from build123d import *

# Parameters (mm, degrees)
SKETCH1_R           = 2.7
BOSS_EXTRUDE1_DEPTH = 5.2
LOWER_THREADS_R     = 6.6
LOWER_THREADS_R_2   = 4.5
BOSS_EXTRUDE2_DEPTH = 11.5


with BuildPart() as part:
    # Sketch1 → Boss-Extrude1 (new body)
    with BuildSketch(Plane(origin=(0, 0, 0), x_dir=(1, 0, 0), z_dir=(0, 1, 0))):
        Polygon((8.025168742, 0), (4.012584371, 6.95), (-4.012584371, 6.95), (-8.025168742, 0), (-4.012584371, -6.95), (4.012584371, -6.95), align=None)
        with Locations(Location((0, 0, 0), (0, 0, 270))):
            Circle(SKETCH1_R, mode=Mode.SUBTRACT)
    extrude(amount=-BOSS_EXTRUDE1_DEPTH)

    # Sketch2 → Revolve1 (revolve)
    with BuildSketch(Plane.XY, mode=Mode.PRIVATE) as revolve1_sk:
        Polygon((2.7, 0), (2.7, 25.2), (3.1, 25.2), (3.7, 21), (3.1, 21), (3.7, 15.833333333), (3.1, 15.833333333), (3.7, 10.666666667), (3.1, 10.666666667), (3.7, 5.5), (3.1, 5.5), (3.738709677, 0), align=None)
    revolve(revolve1_sk.sketch.rotate(Axis((0, -1.995266411, 0), (0, 1, 0)), 90), axis=Axis((0, -1.995266411, 0), (0, 1, 0)))

    # Lower Threads → Boss-Extrude2 (add)
    with BuildSketch(Plane.XZ.offset(5.2)):
        with Locations(Location((0, 0, 0), (0, 0, 90))):
            Circle(LOWER_THREADS_R)
        with Locations(Location((0, 0, 0), (0, 0, 90))):
            Circle(LOWER_THREADS_R_2, mode=Mode.SUBTRACT)
    extrude(amount=BOSS_EXTRUDE2_DEPTH)


solid = part.part
Input: part model. Units: mm. Frame: model coordinates. A direction names the side the tool comes from. Coordinates: 2 decimals unless noted, no trailing zeros. Loops run counter-clockwise (first coordinate to the right, second up) from the corner with the lowest first, then second, coordinate; pieces in that order, holes last. Notation, with made-up numbers: (61.5, 17) -> (79.5, 17) arc R21 cw to (79.5, 47) -> close; hole circle Ø7 at (1.5, 3). An arc over 180 degrees is marked (long way). Write item = value, one per line. Start each with the question number.
Item 1: Material intervals for line 1 (Y direction, x = -4.5, z = -3); line 2 (Y direction, x = -4.75, z = 5.25); line 3 (X direction, y = 15.5, z = 0), sorted ascending.
Item 2: Cut plane B-B, the plane z = -5.25. Return loops of the section in (x, y), plus the area to 3 significant figures.
Item 3: Cut plane A-A, the plane y = -14. Return loops of the section in (x, z), plus the area to 3 significant figures.
Item 4: Mould query, pull axis X, two halves, no side actions, for faces 1 (the face through (4.016, -10.87, -5.238)), 2 (the face through (0, -5.2, 3)), 3 (the face through (0, -3, -6.95)). Classes: pulls with the +X half, pulls with the -X half, needs draft (parallel to the pull), parting line crosses it, or undercut.
Item 5: First-contact query: P1, Ø5, axis at y = -8.5, z = 5, coming from the -X side; P2, Ø1.5, axis at x = 0, y = -8.5, coming from the +Z side; P3, Ø2, axis at x = 1, z = -1.5, coming from the -Y side; P4, Ø4.5, axis at x = 0, z = 0, coming from the -Y side. Flat tips, straight axial feed; report the tip coordinate or a pass-through.
Item 6: Reachability of faces 4 (the face through (-1.352, -10.87, 4.292)), 5 (the face through (-0.147, 13.788, 3.334)), 6 (the face through (0, -3, 6.95)) from +Z, -Z, +X, -X, +Y, -Y: full face, straight path, thin tool, end or side. Return the list, or none.
Item 7: Cut plane D-D, the plane y = 9.5. Return loops of the section in (x, z), plus the area to 3 significant figures.
Item 8: Cut plane C-C, the plane x = 5. Return loops of the section in (y, z), plus the area to 3 significant figures.
Ans:
q1.line_1 = -16.7 to 0
q1.line_2 = -5.2 to 0
q1.line_3 = -3.14 to -2.7, 2.7 to 3.14
q2.outline = (-4.99, -5.2) -> (-4, -5.2) -> (-4, -16.7) -> (4, -16.7) -> (4, -5.2) -> (4.99, -5.2) -> (4.99, 0) -> (-4.99, 0) -> close
q2.area = 144 mm²
q3.outline = circle Ø13.2 at (0, 0); hole circle Ø9 at (0, 0)
q3.area = 73.2 mm²
q4.face_1 = parting line crosses it
q4.face_2 = undercut
q4.face_3 = needs draft
q5.P1 = -6.11
q5.P2 = 6.6
q5.P3 = -5.2
q5.P4 = through
q6.face_4 = -Y
q6.face_5 = none
q6.face_6 = +Z, +X, -X, +Y, -Y
q7.outline = circle Ø6.47 at (0, 0); hole circle Ø5.4 at (0, 0)
q7.area = 9.99 mm²
q8.outline = (-16.7, -4.31) -> (-5.2, -4.31) -> (-5.2, -5.24) -> (0, -5.24) -> (0, 5.24) -> (-5.2, 5.24) -> (-5.2, 4.31) -> (-16.7, 4.31) -> close
q8.area = 154 mm²
